```python
from build123d import *

# Parameters (mm, degrees)
SKETCH1_W                = 33.6
SKETCH1_H                = 30
BOSS_EXTRUDE1_DEPTH      = 4
SKETCH3_W                = 33.6
SKETCH3_H                = 3
BOSS_EXTRUDE2_DEPTH      = 39.2
SKETCH5_W                = 14
SKETCH5_H                = 9
CUT_EXTRUDE2_DEPTH       = 30
SKETCH8_W                = 12
SKETCH8_H                = 7
CUT_EXTRUDE4_DEPTH       = 46.20929108
SKETCH10_W               = 2
SKETCH10_H               = 7.5
BOSS_EXTRUDE3_DEPTH      = 24.3
SKETCH12_W               = 4
SKETCH12_H               = 30
BOSS_EXTRUDE4_DEPTH      = 5
SKETCH13_W               = 2.5
SKETCH13_H               = 8
CUT_EXTRUDE5_DEPTH       = 48.295665763
FILLET3_R                = 0.25
FILLET4_R                = 1
CUT_EXTRUDE6_REACH       = 58.747
SKETCH15_R               = 1.75
FILLET6_R                = 3.75
CUT_EXTRUDE8_REACH       = 49.296
SKETCH23_R               = 1.25
FILLET8_R                = 2
CUT_EXTRUDE9_REACH       = 58.934
SKETCH24_W               = 12
SKETCH24_H               = 18
ESBO_O1_W                = 7.49
ESBO_O1_H                = 3
RESSALTO_EXTRUS_O1_DEPTH = 5.475
FILETE1_R                = 3.7338
FILETE2_R                = 3.7338
ESBO_O2_R                = 1.7
CORTE_EXTRUS_O1_DEPTH    = 5
ESBO_O3_W                = 6.66
ESBO_O3_H                = 2
RESSALTO_EXTRUS_O2_DEPTH = 10.8
CORTE_EXTRUS_O2_REACH    = 54.114
ESBO_O5_R                = 1.7
FILETE3_R                = 3.33
FILETE4_R                = 3.33
FILLET3_OF_ESPELHAR5_R   = 0.25
FILLET6_OF_ESPELHAR5_R   = 3.75
FILLET8_OF_ESPELHAR5_R   = 2
FILETE1_OF_ESPELHAR5_R   = 3.7338
FILETE2_OF_ESPELHAR5_R   = 3.7338
FILETE3_OF_ESPELHAR5_R   = 3.33
FILETE4_OF_ESPELHAR5_R   = 3.33


with BuildPart() as part:
    # Sketch1 → Boss-Extrude1 (new body)
    with BuildSketch(Plane.XY):
        Rectangle(SKETCH1_W, SKETCH1_H)
    extrude(amount=BOSS_EXTRUDE1_DEPTH)

    # Sketch3 → Boss-Extrude2 (add)
    with BuildSketch(Plane.XY.offset(4)):
        with Locations((0, 13.5)):
            Rectangle(SKETCH3_W, SKETCH3_H)
    extrude(amount=BOSS_EXTRUDE2_DEPTH)

    # Sketch5 → Cut-Extrude2 (cut)
    with BuildSketch(Plane.XY.offset(4)):
        with Locations((0, -3.55)):
            Rectangle(SKETCH5_W, SKETCH5_H)
    extrude(amount=-CUT_EXTRUDE2_DEPTH, mode=Mode.SUBTRACT)

    # Sketch8 → Cut-Extrude4 (cut, through all)
    with BuildSketch(Plane.XY.offset(4)):
        with Locations((0, 8.5)):
            Rectangle(SKETCH8_W, SKETCH8_H)
    extrude(amount=-CUT_EXTRUDE4_DEPTH, mode=Mode.SUBTRACT)

    # Sketch10 → Boss-Extrude3 (add)
    with BuildSketch(Plane.XZ.offset(-12)):
        with Locations((15.8, 39.45)):
            Rectangle(SKETCH10_W, SKETCH10_H)
    boss_extrude3 = extrude(amount=BOSS_EXTRUDE3_DEPTH)

    # Sketch12 → Boss-Extrude4 (add)
    with BuildSketch(Plane(origin=(16.8, 0, 0), x_dir=(0, 0, -1), z_dir=(1, 0, 0))):
        with Locations((-2, 0)):
            Rectangle(SKETCH12_W, SKETCH12_H)
    boss_extrude4 = extrude(amount=BOSS_EXTRUDE4_DEPTH)

    # Sketch13 → Cut-Extrude5 (cut, through all)
    with BuildSketch(Plane.XY.offset(4)):
        with Locations((17.55, -8.475)):
            Rectangle(SKETCH13_W, SKETCH13_H)
    cut_extrude5 = extrude(amount=-CUT_EXTRUDE5_DEPTH, mode=Mode.SUBTRACT)

    # Fillet3
    fillet3_edges = [part.edges().sort_by_distance(p)[0] for p in [
        (18.8, -4.475, 2),
        (18.8, -12.475, 2),
        (16.3, -12.475, 2),
        (16.3, -4.475, 2),
    ]]
    fillet(fillet3_edges, radius=FILLET3_R)

    # Fillet4
    fillet4_edges = [part.edges().sort_by_distance(p)[0] for p in [
        (7, 0.95, 2),
        (7, -8.05, 2),
        (-7, -8.05, 2),
        (-7, 0.95, 2),
        (6, 5, 2),
        (-6, 5, 2),
    ]]
    fillet(fillet4_edges, radius=FILLET4_R)

    # Sketch15 → Cut-Extrude6 (cut, up to next)
    with BuildSketch(Plane(origin=(16.8, 0, 0), x_dir=(0, 0, -1), z_dir=(1, 0, 0)), mode=Mode.PRIVATE) as cut_extrude6_sk1:
        with Locations((-39.45, -8.475)):
            Circle(SKETCH15_R)
    cut_extrude6_tool1 = extrude(cut_extrude6_sk1.sketch, amount=-CUT_EXTRUDE6_REACH, mode=Mode.PRIVATE) & part.part
    cut_extrude6 = cut_extrude6_tool1.solids().sort_by_distance((16.8, -8.475, 39.45))[0]
    add(cut_extrude6, mode=Mode.SUBTRACT)

    # Fillet6
    fillet6_edges = [part.edges().sort_by_distance(p)[0] for p in [
        (15.8, -12.3, 35.7),
        (15.8, -12.3, 43.2),
    ]]
    fillet(fillet6_edges, radius=FILLET6_R - 0.0001)  # a hair under: the kernel refuses the full size

    # Sketch23 → Cut-Extrude8 (cut, up to next)
    with BuildSketch(Plane.XY.offset(4), mode=Mode.PRIVATE) as cut_extrude8_sk1:
        with Locations((11.4, -12.5)):
            Circle(SKETCH23_R)
    cut_extrude8_tool1 = extrude(cut_extrude8_sk1.sketch, amount=-CUT_EXTRUDE8_REACH, mode=Mode.PRIVATE) & part.part
    # Sketch23 → Cut-Extrude8 (cut, up to next)
    with BuildSketch(Plane.XY.offset(4), mode=Mode.PRIVATE) as cut_extrude8_sk2:
        with Locations((19.3, 12.5)):
            Circle(SKETCH23_R)
    cut_extrude8_tool2 = extrude(cut_extrude8_sk2.sketch, amount=-CUT_EXTRUDE8_REACH, mode=Mode.PRIVATE) & part.part
    cut_extrude8_1 = cut_extrude8_tool1.solids().sort_by_distance((11.4, -12.5, 4))[0]
    add(cut_extrude8_1, mode=Mode.SUBTRACT)
    cut_extrude8_2 = cut_extrude8_tool2.solids().sort_by_distance((19.3, 12.5, 4))[0]
    add(cut_extrude8_2, mode=Mode.SUBTRACT)
    cut_extrude8 = cut_extrude8_1 + cut_extrude8_2  # Cut-Extrude8 as one shape, for the pattern or mirror that repeats it

    # Fillet8
    fillet8_edges = [part.edges().sort_by_distance(p)[0] for p in [
        (21.8, 15, 2),
        (21.8, -15, 2),
    ]]
    fillet(fillet8_edges, radius=FILLET8_R)

    # Sketch24 → Cut-Extrude9 (cut, up to next)
    with BuildSketch(Plane(origin=(0, 15, 0), x_dir=(1, 0, 0), z_dir=(0, 1, 0)), mode=Mode.PRIVATE) as cut_extrude9_sk1:
        Rectangle(SKETCH24_W, SKETCH24_H)
    cut_extrude9_tool1 = extrude(cut_extrude9_sk1.sketch, amount=-CUT_EXTRUDE9_REACH, mode=Mode.PRIVATE) & part.part
    add(cut_extrude9_tool1.solids().sort_by_distance((0, 15, 0))[0], mode=Mode.SUBTRACT)

    # Esboço1 → Ressalto-extrusão1 (add)
    with BuildSketch(Plane(origin=(16.8, 0, 0), x_dir=(0, 0, -1), z_dir=(1, 0, 0))):
        with Locations((-23.555, 13.5)):
            Rectangle(ESBO_O1_W, ESBO_O1_H)
    ressalto_extrus_o1 = extrude(amount=RESSALTO_EXTRUS_O1_DEPTH)

    # Filete1
    filete1_edges = [part.edges().sort_by_distance(p)[0] for p in [
        (22.275, 13.5, 27.3),
    ]]
    fillet(filete1_edges, radius=FILETE1_R)

    # Filete2
    filete2_edges = [part.edges().sort_by_distance(p)[0] for p in [
        (22.275, 13.5, 19.81),
    ]]
    fillet(filete2_edges, radius=FILETE2_R)

    # Esboço2 → Corte-extrusão1 (cut)
    with BuildSketch(Plane(origin=(0, 15, 0), x_dir=(1, 0, 0), z_dir=(0, 1, 0))):
        with Locations(Location((18.385, -23.39, 0), (0, 0, 270))):
            Circle(ESBO_O2_R)
    corte_extrus_o1 = extrude(amount=-CORTE_EXTRUS_O1_DEPTH, mode=Mode.SUBTRACT)

    # Esboço3 → Ressalto-extrusão2 (add)
    with BuildSketch(Plane.XY.offset(4)):
        with Locations((18.47, 2.8)):
            Rectangle(ESBO_O3_W, ESBO_O3_H)
    ressalto_extrus_o2 = extrude(amount=RESSALTO_EXTRUS_O2_DEPTH)

    # Esboço5 → Corte-extrusão2 (cut, up to next)
    with BuildSketch(Plane(origin=(0, 3.8, 0), x_dir=(1, 0, 0), z_dir=(0, 1, 0)), mode=Mode.PRIVATE) as corte_extrus_o2_sk1:
        with Locations(Location((18.47, -10.875, 0), (0, 0, 180))):
            Circle(ESBO_O5_R)
    corte_extrus_o2_tool1 = extrude(corte_extrus_o2_sk1.sketch, amount=-CORTE_EXTRUS_O2_REACH, mode=Mode.PRIVATE) & part.part
    corte_extrus_o2 = corte_extrus_o2_tool1.solids().sort_by_distance((18.47, 3.8, 10.875))[0]
    add(corte_extrus_o2, mode=Mode.SUBTRACT)

    # Filete3
    filete3_edges = [part.edges().sort_by_distance(p)[0] for p in [
        (21.8, 2.8, 14.8),
    ]]
    fillet(filete3_edges, radius=FILETE3_R)

    # Filete4
    filete4_edges = [part.edges().sort_by_distance(p)[0] for p in [
        (15.14, 2.8, 14.8),
    ]]
    fillet(filete4_edges, radius=FILETE4_R - 0.0001)  # a hair under: the kernel refuses the full size

    # Espelhar5: Boss-Extrude3, Boss-Extrude4, Cut-Extrude5, Cut-Extrude6, Cut-Extrude8, Ressalto-extrusão1, Corte-extrusão1, Ressalto-extrusão2, Corte-extrusão2 across plane
    add(boss_extrude3.mirror(Plane.ZY))
    add(boss_extrude4.mirror(Plane.ZY))
    add(cut_extrude5.mirror(Plane.ZY), mode=Mode.SUBTRACT)
    add(cut_extrude6.mirror(Plane.ZY), mode=Mode.SUBTRACT)
    add(cut_extrude8.mirror(Plane.ZY), mode=Mode.SUBTRACT)
    add(ressalto_extrus_o1.mirror(Plane.ZY))
    add(corte_extrus_o1.mirror(Plane.ZY), mode=Mode.SUBTRACT)
    add(ressalto_extrus_o2.mirror(Plane.ZY))
    add(corte_extrus_o2.mirror(Plane.ZY), mode=Mode.SUBTRACT)

    # Fillet3 of Espelhar5
    fillet3_of_espelhar5_edges = [part.edges().sort_by_distance(p)[0] for p in [
        (-18.8, -4.475, 2),
        (-18.8, -12.475, 2),
        (-16.3, -12.475, 2),
        (-16.3, -4.475, 2),
    ]]
    fillet(fillet3_of_espelhar5_edges, radius=FILLET3_OF_ESPELHAR5_R)

    # Fillet6 of Espelhar5
    fillet6_of_espelhar5_edges = [part.edges().sort_by_distance(p)[0] for p in [
        (-15.8, -12.3, 35.7),
        (-15.8, -12.3, 43.2),
    ]]
    fillet(fillet6_of_espelhar5_edges, radius=FILLET6_OF_ESPELHAR5_R - 0.0001)  # a hair under: the kernel refuses the full size

    # Fillet8 of Espelhar5
    fillet8_of_espelhar5_edges = [part.edges().sort_by_distance(p)[0] for p in [
        (-21.8, 15, 2),
        (-21.8, -15, 2),
    ]]
    fillet(fillet8_of_espelhar5_edges, radius=FILLET8_OF_ESPELHAR5_R)

    # Filete1 of Espelhar5
    filete1_of_espelhar5_edges = [part.edges().sort_by_distance(p)[0] for p in [
        (-22.275, 13.5, 27.3),
    ]]
    fillet(filete1_of_espelhar5_edges, radius=FILETE1_OF_ESPELHAR5_R)

    # Filete2 of Espelhar5
    filete2_of_espelhar5_edges = [part.edges().sort_by_distance(p)[0] for p in [
        (-22.275, 13.5, 19.81),
    ]]
    fillet(filete2_of_espelhar5_edges, radius=FILETE2_OF_ESPELHAR5_R)

    # Filete3 of Espelhar5
    filete3_of_espelhar5_edges = [part.edges().sort_by_distance(p)[0] for p in [
        (-21.8, 2.8, 14.8),
    ]]
    fillet(filete3_of_espelhar5_edges, radius=FILETE3_OF_ESPELHAR5_R)

    # Filete4 of Espelhar5
    filete4_of_espelhar5_edges = [part.edges().sort_by_distance(p)[0] for p in [
        (-15.14, 2.8, 14.8),
    ]]
    fillet(filete4_of_espelhar5_edges, radius=FILETE4_OF_ESPELHAR5_R - 0.0001)  # a hair under: the kernel refuses the full size


solid = part.part
```
Source: CAD feature listing. Evaluate the final solid. Frame: model axes, mm. A direction names the side the tool comes from. Round coordinates to 2 decimals unless told otherwise and drop trailing zeros. Loops run counter-clockwise (first coordinate to the right, second up) from the corner with the lowest first, then second, coordinate; pieces in that order, holes last. Notation, with made-up numbers: M -37,58.5 L 7,58.5 A20 ccw 7,63.5 Z; hole C -7,52.5 d5. An arc over 180 degrees is marked long. Use a Markdown table: item, result. Add a question column.
1. Cut plane B-B, the plane y = -2.75. Output: boundary loops of the cut face in (x, z).
2. Set-up query: faces 4 (the flat face through (18, 1.8, 8)), 5 (the flat face through (16.8, 5, 39)), 6 (the flat face through (-14.8, 0, 39)). Return all of +Z, -Z, +X, -X, +Y, -Y with unobstructed straight access to the full face (end or side cutting, diameter ignored); none if empty.
3. Cut plane C-C, the plane x = -11.4. Output: boundary loops of the cut face in (y, z), and give its area (3 significant figures).
4. Contact query for flat-ended pins moving along their axis: pin 1 (7.5 mm diameter, centred on x = 18, z = 10, fed in from -Y); pin 2 (10 mm diameter, centred on y = 8.5, z = 6, fed in from -X); pin 3 (4 mm diameter, centred on x = -18.385, z = 23.39, fed in from -Y). Output: stop coordinate, or through.
5. Pull-direction query (X, two-part tool) for faces 1 (the cylindrical face through (-16.14, 2.81, 13.85)), 2 (the cylindrical face through (21.15, 13.52, 26.24)), 3 (the flat face through (18, 3.8, 8)); classes: +X half, -X half, draft (parallel to the pull), parting line (faces both ways), or undercut.
6. Cut plane D-D, the plane x = 12. Output: boundary loops of the cut face in (y, z).
7. Cut plane A-A, the plane x = 4. Output: boundary loops of the cut face in (y, z).
8. Ray query, line 1 along X through (y, z) = (14.3, 23.39) (3 decimals); line 2 along Z through (x, y) = (-18.47, 2.7) (3 decimals); line 3 along Z through (x, y) = (15, -7.5). Return the intervals inside material, ascending. Write a range as [from, to].
Solution:
| question | item | result |
|---|---|---|
| 1 | outline | M -21.8,0 L -7,0 L -7,4 L -21.8,4 Z; M -16.8,35.7 L -14.8,35.7 L -14.8,43.2 L -16.8,43.2 Z; M 7,0 L 21.8,0 L 21.8,4 L 7,4 Z; M 14.8,35.7 L 16.8,35.7 L 16.8,43.2 L 14.8,43.2 Z |
| 2 | face 4 | +X, -X, -Y |
| 2 | face 5 | +Z, +X, +Y, -Y |
| 2 | face 6 | +Z, -Y |
| 3 | outline | M -15,0 L -13.75,0 L -13.75,4 L -15,4 Z; M -11.25,0 L 15,0 L 15,43.2 L 12,43.2 L 12,4 L -11.25,4 Z |
| 3 | area | 228 mm2 |
| 4 | pin 1 | stops at y = 1.8 |
| 4 | pin 2 | stops at x = -21.8 |
| 4 | pin 3 | stops at y = 12 |
| 5 | face 1 | undercut |
| 5 | face 2 | +X half |
| 5 | face 3 | draft |
| 6 | outline | M -15,0 L -13.6,0 L -13.6,4 L -15,4 Z; M -11.4,0 L 15,0 L 15,43.2 L 12,43.2 L 12,4 L -11.4,4 Z |
| 7 | outline | M -15,0 L -8.05,0 L -8.05,4 L -15,4 Z; M 0.95,0 L 5,0 L 5,4 L 0.95,4 Z; M 12,9 L 15,9 L 15,43.2 L 12,43.2 Z |
| 8 | line 1 | x = [-22.272, -20.085], [-16.685, 16.685], [20.085, 22.272] |
| 8 | line 2 | z = [0, 9.175], [12.575, 14.8] |
| 8 | line 3 | z = [0, 4], [35.7, 38], [40.9, 43.2] |
